Work out the finished part from the listing and answer in its coordinate system (mm). A direction names the side the tool comes from. Coordinates: 2 decimals unless noted, no trailing zeros. Write each loop counter-clockwise with the first axis right and the second up, starting at its lowest first coordinate (ties: lowest second). Pieces come first, ordered by that corner, then holes. Notation, with made-up numbers: (-37.75, 60.5) - (15.25, 60.5) arc R18 ccw to (15.25, 84.5) - close; hole circle Ø2 at (-17.75, -27). An arc over 180 degrees is marked (long way). Use one line per item in the form item = value. Start each with the question number.
Item 1: For faces 1 (the cylindrical face through (-7.94, 2.48, 8.58)), 2 (the flat face through (-10.77, 1.46, 8.54)), 3 (the flat face through (0, 2.725, 6)), determine the directions among +Z, -Z, +X, -X, +Y, -Y from which every point of the face is accessible in a straight line to the end or side of a thin tool.
Item 2: A cutting plane is placed at D-D (y = 1.75). Write down the section's boundary in (x, z).
Item 3: Consider probe 1 along X at (y, z) = (1, 7.5); probe 2 along X at (y, z) = (1.55, 6.5); probe 3 along Z at (x, y) = (-11.25, 12.25). Determine where each line is inside the solid, lowest interval first.
Item 4: Determine the mould class of faces 4 (the cylindrical face through (8.08, 9.62, 0.99)), 5 (the flat face through (10.845, 1.458, 8.465)), 6 (the flat face through (0, 9, 0)) for opening direction X: released by +X, released by -X, zero draft, split by the parting line, or undercut.
Item 5: A cutting plane is placed at C-C (y = 10). Write down the section's boundary in (x, z).
Item 6: A cutting plane is placed at B-B (z = 7). Write down the section's boundary in (x, y).
Item 7: A cutting plane is placed at A-A (y = 6.25). Write down the section's boundary in (x, z).
Item 8: Given pin 1 (10 mm diameter, centred on x = 8, y = 14.5, fed in from +Z); pin 2 (1.3 mm diameter, centred on x = -8, z = 6, fed in from +Y); pin 3 (5 mm diameter, centred on x = 7.5, z = 7.5, fed in from +Y), each flat-ended and moving along its own axis, determine where each tip first touches the part or whether it passes through.
from build123d import *

# Parameters (mm, degrees)
SKETCH1_R           = 1.25
BOSS_EXTRUDE1_DEPTH = 2
SKETCH2_W           = 26.619471542
SKETCH2_H           = 2.5
BOSS_EXTRUDE2_DEPTH = 9
SKETCH3_R           = 1.25
CUT_EXTRUDE1_DEPTH  = 9
SKETCH4_R           = 2.25
CUT_EXTRUDE2_DEPTH  = 0.5
CHAMFER1_SIZE       = 5


with BuildPart() as part:
    # Sketch1 → Boss-Extrude1 (new body)
    with BuildSketch(Plane.XY):
        with BuildLine():
            Line((-13.309735771, 0.225207445), (13.309735771, 0.225207445))
            Line((13.309735771, 0.225207445), (13.309735771, 8.907396156))
            ThreePointArc((13.309735771, 8.907396156), (12.953344247, 10.761284051), (11.934975641, 12.350887972))
            ThreePointArc((11.934975641, 12.350887972), (0, 17.475207445), (-11.934975641, 12.350887972))
            ThreePointArc((-11.934975641, 12.350887972), (-12.953344247, 10.761284051), (-13.309735771, 8.907396156))
            Line((-13.309735771, 8.907396156), (-13.309735771, 0.225207445))
        make_face()
        with Locations((7.499735771, 10.725207445)):
            Circle(SKETCH1_R, mode=Mode.SUBTRACT)
        with Locations((-7.500264229, 10.725207445)):
            Circle(SKETCH1_R, mode=Mode.SUBTRACT)
        with Locations((-0.000264229, 5.725207445)):
            Circle(SKETCH1_R, mode=Mode.SUBTRACT)
    extrude(amount=BOSS_EXTRUDE1_DEPTH)

    # Sketch2 → Boss-Extrude2 (add)
    with BuildSketch(Plane.XY.offset(2)):
        with Locations((0, 1.475207445)):
            Rectangle(SKETCH2_W, SKETCH2_H)
    extrude(amount=BOSS_EXTRUDE2_DEPTH)

    # Sketch3 → Cut-Extrude1 (cut)
    with BuildSketch(Plane(origin=(0, 2.725207445, 0), x_dir=(1, 0, 0), z_dir=(0, 1, 0))):
        with Locations(Location((-7.077404832, -6.5, 0), (0, 0, 270))):  # turned: the seam where the file's is
            Circle(SKETCH3_R)
        with Locations(Location((7.077404832, -6.5, 0), (0, 0, 270))):  # turned: the seam where the file's is
            Circle(SKETCH3_R)
    extrude(amount=-CUT_EXTRUDE1_DEPTH, mode=Mode.SUBTRACT)

    # Sketch4 → Cut-Extrude2 (cut)
    with BuildSketch(Plane(origin=(0, 2.725207445, 0), x_dir=(1, 0, 0), z_dir=(0, 1, 0))):
        with Locations(Location((-7.077404832, -6.5, 0), (0, 0, 270))):  # turned: the seam where the file's is
            Circle(SKETCH4_R)
        with Locations(Location((7.077404832, -6.5, 0), (0, 0, 270))):  # turned: the seam where the file's is
            Circle(SKETCH4_R)
    extrude(amount=-CUT_EXTRUDE2_DEPTH, mode=Mode.SUBTRACT)

    # Chamfer1
    chamfer1_edges = [part.edges().sort_by_distance(p)[0] for p in [
        (13.309735771, 1.475207445, 11),
        (-13.309735771, 1.475207445, 11),
    ]]
    chamfer(chamfer1_edges, length=CHAMFER1_SIZE)


solid = part.part
Answer:
q1.face_1 = +Y
q1.face_2 = +Z, -X, +Y, -Y
q1.face_3 = +Z, +X, -X, +Y
q2.outline = (-13.31, 0) - (13.31, 0) - (13.31, 6) - (8.31, 11) - (-8.31, 11) - (-13.31, 6) - close; hole circle Ø2.5 at (-7.08, 6.5); hole circle Ø2.5 at (7.08, 6.5)
q3.probe_1 = -11.81 to -7.83, -6.33 to 6.33, 7.83 to 11.81
q3.probe_2 = -12.81 to -8.33, -5.83 to 5.83, 8.33 to 12.81
q3.probe_3 = 0 to 2
q4.face_4 = undercut
q4.face_5 = released by +X
q4.face_6 = zero draft
q5.outline = (-13.19, 0) - (-8.52, 0) - (-8.52, 2) - (-13.19, 2) - close; (-6.48, 0) - (6.48, 0) - (6.48, 2) - (-6.48, 2) - close; (8.52, 0) - (13.19, 0) - (13.19, 2) - (8.52, 2) - close
q6.outline = (-12.31, 0.23) - (-8.22, 0.23) - (-8.22, 2.23) - (-9.27, 2.23) - (-9.27, 2.73) - (-12.31, 2.73) - close; (-5.93, 0.23) - (5.93, 0.23) - (5.93, 2.23) - (4.88, 2.23) - (4.88, 2.73) - (-4.88, 2.73) - (-4.88, 2.23) - (-5.93, 2.23) - close; (8.22, 0.23) - (12.31, 0.23) - (12.31, 2.73) - (9.27, 2.73) - (9.27, 2.23) - (8.22, 2.23) - close
q7.outline = (-13.31, 0) - (-1.13, 0) - (-1.13, 2) - (-13.31, 2) - close; (1.13, 0) - (13.31, 0) - (13.31, 2) - (1.13, 2) - close
q8.pin_1 = 2
q8.pin_2 = 2.23
q8.pin_3 = 2.73
